Geometry: see drawing. Coordinates: mm, zero at the bounding-box minimum. A direction names the side the tool comes from. Give positions to 0.01 mm unless a question says otherwise; leave off trailing zeros. Loops run counter-clockwise (first coordinate to the right, second up) from the corner with the lowest first, then second, coordinate; pieces in that order, holes last. Notation, with made-up numbers: M 50.5,-14.75 L 105.5,-14.75 A26 cw 105.5,19.25 Z; hole C 17.5,25 d9. An arc over 180 degrees is marked long. Put each result on its own line as item: value.
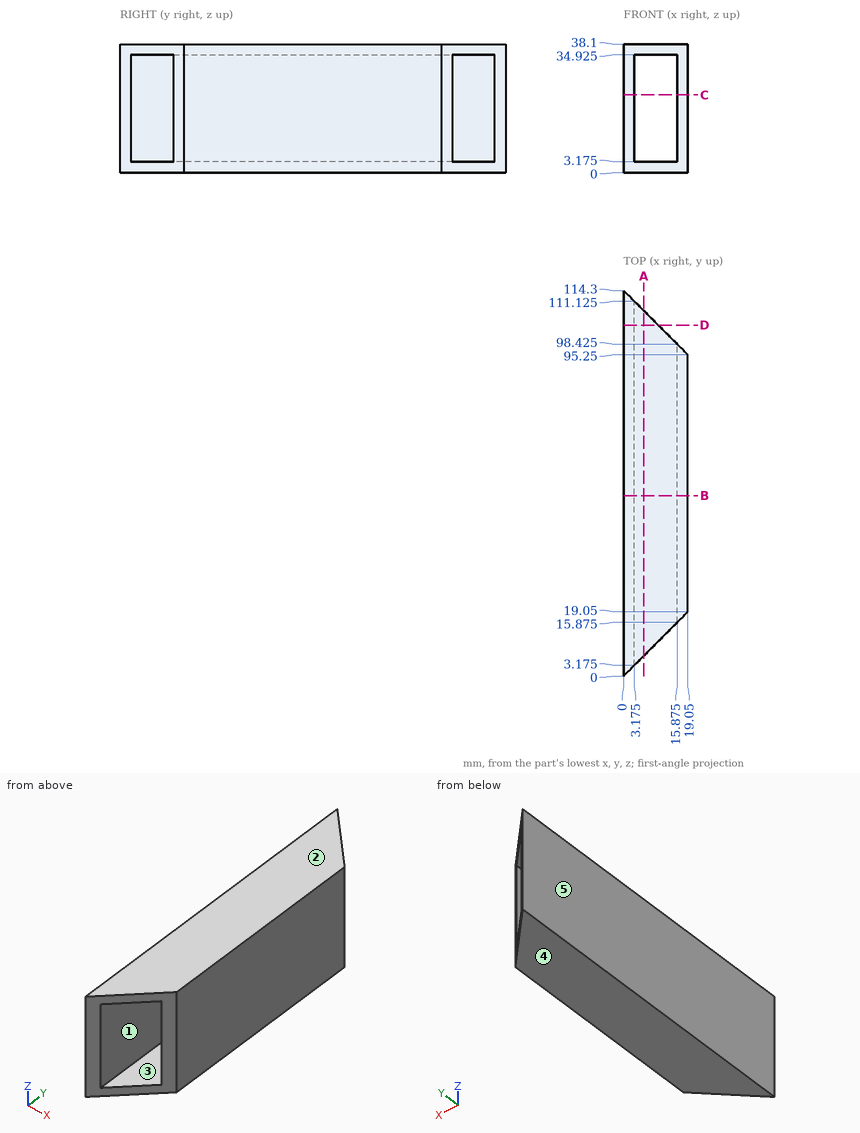
1. Draft query along X for the marked faces 3, 4 and 5. Return one class per face: pulls with the +X half, pulls with the -X half, needs draft (parallel to the pull), parting line crosses it, or undercut.
Found:
face 3: undercut
face 4: needs draft
face 5: pulls with the -X half
2. Section query C-C (z = 23). Output: boundary loops of the cut face in (x, y) (3 decimals).
Found:
outline: M 0,0 L 3.175,3.175 L 3.175,111.125 L 0,114.3 Z; M 15.875,15.875 L 19.05,19.05 L 19.05,95.25 L 15.875,98.425 Z
3. Section query D-D (y = 104). Output: boundary loops of the cut face in (x, z) (3 decimals).
Found:
outline: M 0,0 L 10.3,0 L 10.3,3.175 L 3.175,3.175 L 3.175,34.925 L 10.3,34.925 L 10.3,38.1 L 0,38.1 Z
4. Contact query for a flat-ended pin moving along its axis: P1, Ø6, axis at x = 4, z = 9.5, coming from the +Y side. Output: stop coordinate, or through.
Found:
P1: y = 113.3
5. Material intervals for line 1 (X direction, y = 72, z = 9.5) (3 decimals); line 2 (Z direction, x = 14, y = 36.5) (3 decimals); line 3 (X direction, y = 97, z = 6) (3 decimals), sorted ascending. Write a range as from..to.
Found:
line 1: 0..3.175, 15.875..19.05
line 2: 0..3.175, 34.925..38.1
line 3: 0..3.175, 15.875..17.3
6. Section query A-A (x = 6). Output: boundary loops of the cut face in (y, z) (3 decimals), plus the area to 3 significant figures.
Found:
outline: M 6,0 L 108.3,0 L 108.3,3.175 L 6,3.175 Z; M 6,34.925 L 108.3,34.925 L 108.3,38.1 L 6,38.1 Z
area: 650 mm^2
7. Section query B-B (y = 53.5). Output: boundary loops of the cut face in (x, z) (3 decimals).
Found:
outline: M 0,0 L 19.05,0 L 19.05,38.1 L 0,38.1 Z; hole M 3.175,3.175 L 15.875,3.175 L 15.875,34.925 L 3.175,34.925 Z
8. Access query for the marked faces 1 and 2. Directions: +Z, -Z, +X, -X, +Y, -Y. A direction counts if a zero-diameter tool reaches every point of the face in a straight line with its end or side. Return the directions, or none.
Found:
face 1: +Y, -Y
face 2: +Z, +X, -X, +Y, -Y
